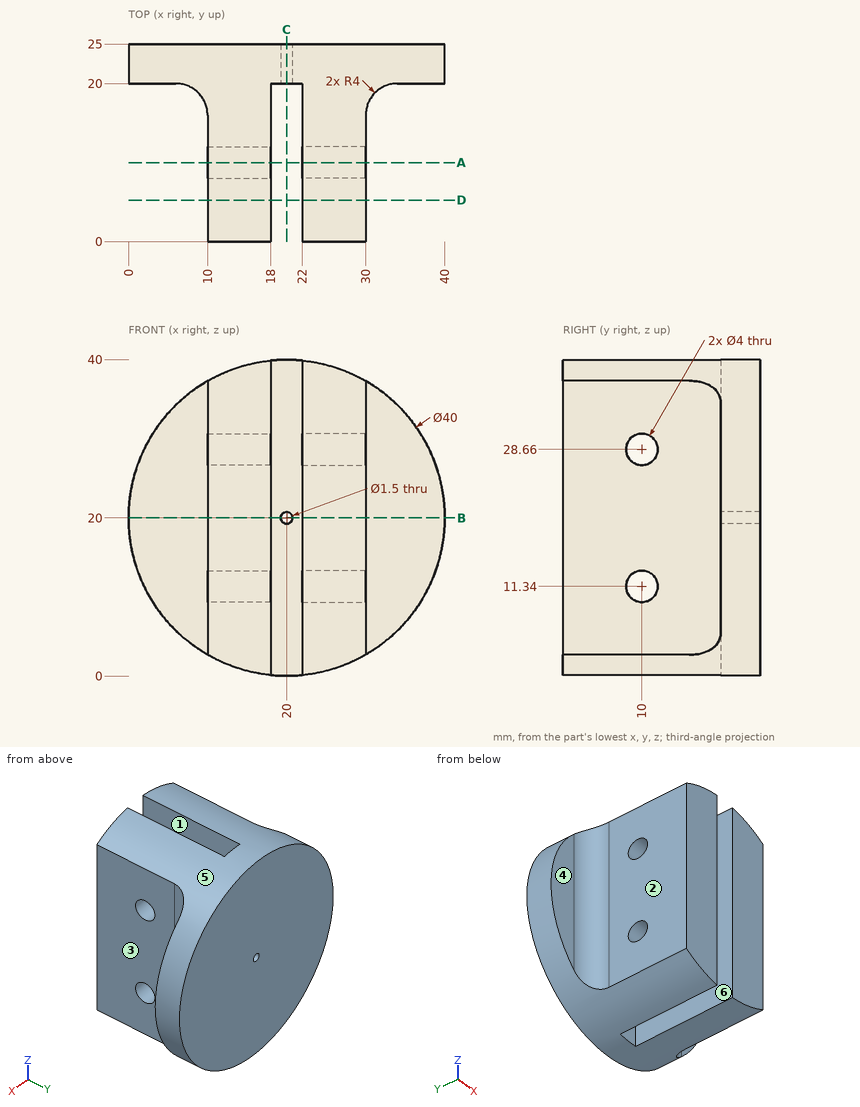
Geometry: see drawing. Coordinates: mm, zero at the bounding-box minimum. A direction names the side the tool comes from. Round coordinates to 2 decimals unless told otherwise and drop trailing zeros. Loops run counter-clockwise (first coordinate to the right, second up) from the corner with the lowest first, then second, coordinate; pieces in that order, holes last. Notation, with made-up numbers: (-39.75, 44.5) -> (-18.75, 44.5) arc R35 ccw to (-18.75, 77.5) -> close; hole circle Ø5 at (-26.75, 20). An arc over 180 degrees is marked (long way). Use one line per item in the form item = value. Start each with the question number.
Item 1: Section query B-B on z = 20. Return the cut outline in (x, y), then the cut area to 3 significant figures.
Item 2: Material intervals for L1, parallel to X at y = 6.5, z = 31; L2, parallel to Y at x = 23, z = 28.5; L3, parallel to Y at x = 35, z = 18, sorted ascending. Write a range as from..to.
Item 3: Mould query, pull axis X, two halves, no side actions, for the marked faces 4, 5 and 6. Classes: pulls with the +X half, pulls with the -X half, needs draft (parallel to the pull), parting line crosses it, or undercut.
Item 4: Section query D-D on y = 5.25. Return the cut outline in (x, z).
Item 5: Section query C-C on x = 20. Return the cut outline in (y, z).
Item 6: Set-up query: the marked faces 1, 2 and 3. Return all of +Z, -Z, +X, -X, +Y, -Y with unobstructed straight access to the full face (end or side cutting, diameter ignored); none if empty.
Item 7: Contact query for flat-ended pins moving along their axis: pin 1 Ø3.5 at (y, z) = (10, 28.66) entering from -X; pin 2 Ø5 at (y, z) = (6.5, 12) entering from +X; pin 3 Ø1 at (y, z) = (5, 17) entering from -X; pin 4 Ø1.8 at (x, z) = (37.5, 18) entering from -Y. Output: stop coordinate, or through.
Item 8: Section query A-A on y = 10. Return the cut outline in (x, z).
Ans:
q1.outline = (0, 20) -> (6, 20) arc R4 cw to (10, 16) -> (10, 0) -> (18, 0) -> (18, 20) -> (19.25, 20) -> (19.25, 25) -> (0, 25) -> close; (20.75, 20) -> (22, 20) -> (22, 0) -> (30, 0) -> (30, 16) arc R4 cw to (34, 20) -> (40, 20) -> (40, 25) -> (20.75, 25) -> close
q1.area = 519 mm^2
q2.L1 = 10..18, 22..30
q2.L2 = 0..8.01, 11.99..25
q2.L3 = 20..25
q3.face_4 = needs draft
q3.face_5 = parting line crosses it
q3.face_6 = undercut
q4.outline = (10, 2.68) arc R20 ccw to (18, 0.1) -> (18, 39.9) arc R20 ccw to (10, 37.32) -> close; (22, 0.1) arc R20 ccw to (30, 2.68) -> (30, 37.32) arc R20 ccw to (22, 39.9) -> close
q5.outline = (20, 0) -> (25, 0) -> (25, 19.25) -> (20, 19.25) -> close; (20, 20.75) -> (25, 20.75) -> (25, 40) -> (20, 40) -> close
q6.face_1 = +Z, -Z, -Y
q6.face_2 = +Z, -Z, -X, -Y
q6.face_3 = +Z, -Z, +X, -Y
q7.pin_1 = through
q7.pin_2 = 30
q7.pin_3 = 10
q7.pin_4 = 20
q8.outline = (10, 2.68) arc R20 ccw to (18, 0.1) -> (18, 9.34) -> (10, 9.34) -> close; (10, 13.34) -> (18, 13.34) -> (18, 26.66) -> (10, 26.66) -> close; (10, 30.66) -> (18, 30.66) -> (18, 39.9) arc R20 ccw to (10, 37.32) -> close; (22, 0.1) arc R20 ccw to (30, 2.68) -> (30, 9.34) -> (22, 9.34) -> close; (22, 13.34) -> (30, 13.34) -> (30, 26.66) -> (22, 26.66) -> close; (22, 30.66) -> (30, 30.66) -> (30, 37.32) arc R20 ccw to (22, 39.9) -> close
